```python
from build123d import *
from build123d.topology import SkipClean

# Parameters (mm, degrees)
BOSS_EXTRUDE1_DEPTH       = 1
BOSS_EXTRUDE1_DEPTH_BACK  = 1
SKETCH1_R                 = 5
SKETCH1_R_2               = 0.5
BOSS_EXTRUDE2_START       = -5.85
BOSS_EXTRUDE2_OUTLINE_W   = 15
BOSS_EXTRUDE2_OUTLINE_H   = 4
BOSS_EXTRUDE2_DEPTH       = 3
BOSS_EXTRUDE2_START_2     = -4
BOSS_EXTRUDE2_2_OUTLINE_R = 0.5
BOSS_EXTRUDE2_2_DEPTH     = 6
CUT_EXTRUDE4_DEPTH        = 8
SKETCH6_R                 = 0.8
CUT_EXTRUDE3_DEPTH        = 9
SKETCH9_W                 = 8
SKETCH9_H                 = 0.25
CUT_EXTRUDE5_DEPTH        = 2
SKETCH10_R                = 2.1
SKETCH10_R_2              = 0.8
CUT_EXTRUDE6_DEPTH        = 1.5
FILLET2_R                 = 1
FILLET3_START             = -5.85
FILLET3_DEPTH             = 1.5
CUT_EXTRUDE2_START        = -10
CUT_EXTRUDE2_DEPTH        = 10
BOSS_EXTRUDE3_START       = -2
BOSS_EXTRUDE3_DEPTH       = 2
FILLET4_R                 = 0.5
CUT_EXTRUDE7_DEPTH        = 1.5


with BuildPart() as part:
    # Sketch1 → Boss-Extrude1 (new, two sides: drawn at the far end of the back side and taken through both)
    with BuildSketch(Plane.XY.offset(-BOSS_EXTRUDE1_DEPTH_BACK)):
        Circle(SKETCH1_R)
        with Locations((-2.5, 1.095)):
            Circle(SKETCH1_R_2, mode=Mode.SUBTRACT)
        with Locations((2.5, 1.095)):
            Circle(SKETCH1_R_2, mode=Mode.SUBTRACT)
        with Locations((-2.5, -1.095)):
            Circle(SKETCH1_R_2, mode=Mode.SUBTRACT)
        with Locations((2.5, -1.095)):
            Circle(SKETCH1_R_2, mode=Mode.SUBTRACT)
        with Locations((-1.35, 2.5)):
            Circle(SKETCH1_R_2, mode=Mode.SUBTRACT)
        with Locations((-1.35, -2.5)):
            Circle(SKETCH1_R_2, mode=Mode.SUBTRACT)
    extrude(amount=BOSS_EXTRUDE1_DEPTH + BOSS_EXTRUDE1_DEPTH_BACK)

    # Boss-Extrude2: read off the stored shape, not the designer's step
    # Boss-Extrude2 outline → Boss-Extrude2 (add)
    with BuildSketch(Plane.YZ.offset(BOSS_EXTRUDE2_START)):
        with Locations((0, -1)):
            Rectangle(BOSS_EXTRUDE2_OUTLINE_W, BOSS_EXTRUDE2_OUTLINE_H)
    extrude(amount=BOSS_EXTRUDE2_DEPTH)

    # Boss-Extrude2 2 outline → Boss-Extrude2 2 (cut)
    with SkipClean():  # the faces are left unmerged after this step: merging them gives an invalid solid
        with BuildSketch(Plane.XY.offset(BOSS_EXTRUDE2_START_2)):
            with Locations((-2.5, 1.095)):
                Circle(BOSS_EXTRUDE2_2_OUTLINE_R)
            with Locations((-2.5, -1.095)):
                Circle(BOSS_EXTRUDE2_2_OUTLINE_R)
        extrude(amount=BOSS_EXTRUDE2_2_DEPTH, mode=Mode.SUBTRACT)

    # Sketch7 → Cut-Extrude4 (cut)
    with SkipClean():  # the faces are left unmerged after this step: merging them gives an invalid solid
        with BuildSketch(Plane(origin=(-2.85, 0, 0), x_dir=(0, 0, -1), z_dir=(1, 0, 0))):
            Polygon((-1, 7.5), (-1, 4.10822346), (1, 4.10822346), (1, 1.452071421), (3, 1.452071421), (3, 7.5), align=None)
            Polygon((-1, -4.10822346), (-1, -7.5), (3, -7.5), (3, -1.452071421), (1, -1.452071421), (1, -4.10822346), align=None)
        extrude(amount=CUT_EXTRUDE4_DEPTH, mode=Mode.SUBTRACT)

    # Sketch6 → Cut-Extrude3 (cut)
    with SkipClean():  # the faces are left unmerged after this step: merging them gives an invalid solid
        with BuildSketch(Plane.ZY.offset(5.85)):
            with Locations(Location((-1, 5.5, 0), (0, 0, 270))):
                Circle(SKETCH6_R)
            with Locations(Location((-1, -5.5, 0), (0, 0, 270))):
                Circle(SKETCH6_R)
        extrude(amount=-CUT_EXTRUDE3_DEPTH, mode=Mode.SUBTRACT)

    # Sketch9 → Cut-Extrude5 (cut)
    with SkipClean():  # the faces are left unmerged after this step: merging them gives an invalid solid
        with BuildSketch(Plane.XY.offset(1)):
            with Locations((1.15, 3.98322346)):
                Rectangle(SKETCH9_W, SKETCH9_H)
            with Locations((1.15, -3.98322346)):
                Rectangle(SKETCH9_W, SKETCH9_H)
        extrude(amount=-CUT_EXTRUDE5_DEPTH, mode=Mode.SUBTRACT)

    # Sketch10 → Cut-Extrude6 (cut)
    # profile 1 of 2: a face of its own
    with SkipClean():  # the faces are left unmerged after this step: merging them gives an invalid solid
        with BuildSketch(Plane.ZY.offset(5.85)):
            with Locations((-1, 5.5)):
                Circle(SKETCH10_R)
            with Locations((-1, 5.5)):
                Circle(SKETCH10_R_2, mode=Mode.SUBTRACT)
        # profile 2 of 2: a face of its own
        with BuildSketch(Plane.ZY.offset(5.85)):
            with Locations((-1, -5.5)):
                Circle(SKETCH10_R)
            with Locations((-1, -5.5)):
                Circle(SKETCH10_R_2, mode=Mode.SUBTRACT)
        extrude(amount=-CUT_EXTRUDE6_DEPTH, mode=Mode.SUBTRACT)

    # Fillet2
    fillet2_edges = [part.edges().sort_by_distance(p)[0] for p in [
        (-4.35, 7.5, -3),
        (-4.35, -7.5, 1),
        (-4.35, -7.5, -3),
        (-4.35, 7.5, 1),
    ]]
    fillet(fillet2_edges, radius=FILLET2_R)

    # Fillet3: read off the stored shape, not the designer's step
    # Fillet3 outline → Fillet3 (cut)
    with SkipClean():  # the faces are left unmerged after this step: merging them gives an invalid solid
        with BuildSketch(Plane.YZ.offset(FILLET3_START)):
            with BuildLine():
                ThreePointArc((-6.696065005, -2.726102113), (-6.574273302, -2.846043449), (-6.5, -3))
                Line((-6.5, -3), (-6.140312424, -3))
                ThreePointArc((-6.140312424, -3), (-6.428345587, -2.883659861), (-6.696065005, -2.726102113))
            make_face()
            with BuildLine():
                ThreePointArc((-7.5, -2), (-7.346043449, -2.074273302), (-7.226102113, -2.196065005))
                ThreePointArc((-7.226102113, -2.196065005), (-7.383659861, -1.928345587), (-7.5, -1.640312424))
                Line((-7.5, -1.640312424), (-7.5, -2))
            make_face()
            with BuildLine():
                ThreePointArc((-3.784723184, -2.211538462), (-4.257978234, -2.693334561), (-4.859687576, -3))
                Line((-4.859687576, -3), (-3.376323942, -3))
                ThreePointArc((-3.376323942, -3), (-3.820300726, -2.729966553), (-3.784723184, -2.211538462))
            make_face()
            with BuildLine():
                Line((-7.5, 0), (-7.5, -0.359687576))
                ThreePointArc((-7.5, -0.359687576), (-7.383659861, -0.071654413), (-7.226102112, 0.196065005))
                ThreePointArc((-7.226102112, 0.196065005), (-7.346043449, 0.074273302), (-7.5, 0))
            make_face()
            with BuildLine():
                ThreePointArc((-4.859687576, 1), (-4.257978234, 0.693334561), (-3.784723184, 0.211538462))
                ThreePointArc((-3.784723184, 0.211538462), (-3.820300726, 0.729966553), (-3.376323942, 1))
                Line((-3.376323942, 1), (-4.859687576, 1))
            make_face()
            with BuildLine():
                ThreePointArc((3.784723184, -2.211538462), (3.820300726, -2.729966553), (3.376323942, -3))
                Line((3.376323942, -3), (4.859687576, -3))
                ThreePointArc((4.859687576, -3), (4.257978234, -2.693334561), (3.784723184, -2.211538462))
            make_face()
            with BuildLine():
                ThreePointArc((-6.5, 1), (-6.574273302, 0.846043449), (-6.696065005, 0.726102113))
                ThreePointArc((-6.696065005, 0.726102113), (-6.428345587, 0.883659861), (-6.140312424, 1))
                Line((-6.140312424, 1), (-6.5, 1))
            make_face()
            with BuildLine():
                Line((4.859687576, 1), (3.376323942, 1))
                ThreePointArc((3.376323942, 1), (3.820300726, 0.729966553), (3.784723184, 0.211538462))
                ThreePointArc((3.784723184, 0.211538462), (4.257978234, 0.693334561), (4.859687576, 1))
            make_face()
            with BuildLine():
                ThreePointArc((6.696065005, -2.726102112), (6.428345587, -2.883659861), (6.140312424, -3))
                Line((6.140312424, -3), (6.5, -3))
                ThreePointArc((6.5, -3), (6.574273302, -2.846043449), (6.696065005, -2.726102112))
            make_face()
            with BuildLine():
                Line((6.5, 1), (6.140312424, 1))
                ThreePointArc((6.140312424, 1), (6.428345587, 0.883659861), (6.696065005, 0.726102112))
                ThreePointArc((6.696065005, 0.726102112), (6.574273302, 0.846043449), (6.5, 1))
            make_face()
            with BuildLine():
                ThreePointArc((7.5, -1.640312424), (7.383659861, -1.928345587), (7.226102112, -2.196065005))
                ThreePointArc((7.226102112, -2.196065005), (7.346043449, -2.074273302), (7.5, -2))
                Line((7.5, -2), (7.5, -1.640312424))
            make_face()
            with BuildLine():
                ThreePointArc((7.5, 0), (7.346043449, 0.074273302), (7.226102113, 0.196065005))
                ThreePointArc((7.226102113, 0.196065005), (7.383659861, -0.071654413), (7.5, -0.359687576))
                Line((7.5, -0.359687576), (7.5, 0))
            make_face()
        extrude(amount=FILLET3_DEPTH, mode=Mode.SUBTRACT)

    # Sketch3 → Cut-Extrude2 (cut)
    with SkipClean():  # the faces are left unmerged after this step: merging them gives an invalid solid
        with BuildSketch(Plane.XY.offset(1).offset(CUT_EXTRUDE2_START)):
            with BuildLine():
                ThreePointArc((3.5, -3.570714214), (5, 0), (3.5, 3.570714214))
                Line((3.5, 3.570714214), (3.5, -3.570714214))
            make_face()
        extrude(amount=CUT_EXTRUDE2_DEPTH, mode=Mode.SUBTRACT)

    # Sketch11 → Boss-Extrude3 (add)
    with SkipClean():  # the faces are left unmerged after this step: merging them gives an invalid solid
        with BuildSketch(Plane.XY.offset(1).offset(BOSS_EXTRUDE3_START)):
            with BuildLine():
                Line((0, -3.85822346), (0, -5))
                ThreePointArc((0, -5), (1.689509204, -4.705906783), (3.180269129, -3.85822346))
                Line((3.180269129, -3.85822346), (0, -3.85822346))
            make_face()
            with BuildLine():
                Line((0, 5), (0, 3.85822346))
                Line((0, 3.85822346), (3.180269129, 3.85822346))
                ThreePointArc((3.180269129, 3.85822346), (1.689509204, 4.705906783), (0, 5))
            make_face()
        extrude(amount=BOSS_EXTRUDE3_DEPTH)

    # Fillet4
    fillet4_edges = [part.edges().sort_by_distance(p)[0] for p in [
        (0, -5, 0),
        (0, -3.85822346, 0),
        (0, 3.85822346, 0),
        (0, 5, 0),
    ]]
    fillet(fillet4_edges, radius=FILLET4_R)

    # Sketch12 → Cut-Extrude7 (cut)
    with BuildSketch(Plane.ZY.offset(5.85)):
        with BuildLine():
            ThreePointArc((1, 6.5), (0.707106781, 7.207106781), (0, 7.5))
            ThreePointArc((0, 7.5), (0.074273302, 7.346043449), (0.196065005, 7.226102113))
            ThreePointArc((0.196065005, 7.226102113), (0.48492424, 6.98492424), (0.726102113, 6.696065005))
            ThreePointArc((0.726102113, 6.696065005), (0.846043449, 6.574273302), (1, 6.5))
        make_face()
        with BuildLine():
            ThreePointArc((-2.726102113, -6.696065005), (-2.48492424, -6.98492424), (-2.196065005, -7.226102113))
            ThreePointArc((-2.196065005, -7.226102113), (-2.074273302, -7.346043449), (-2, -7.5))
            ThreePointArc((-2, -7.5), (-2.707106781, -7.207106781), (-3, -6.5))
            ThreePointArc((-3, -6.5), (-2.846043449, -6.574273302), (-2.726102113, -6.696065005))
        make_face()
        with BuildLine():
            ThreePointArc((0, -7.5), (0.707106781, -7.207106781), (1, -6.5))
            ThreePointArc((1, -6.5), (0.846043449, -6.574273302), (0.726102113, -6.696065005))
            ThreePointArc((0.726102113, -6.696065005), (0.48492424, -6.98492424), (0.196065005, -7.226102113))
            ThreePointArc((0.196065005, -7.226102113), (0.074273302, -7.346043449), (0, -7.5))
        make_face()
        with BuildLine():
            ThreePointArc((-2, 7.5), (-2.707106781, 7.207106781), (-3, 6.5))
            ThreePointArc((-3, 6.5), (-2.846043449, 6.574273302), (-2.726102113, 6.696065005))
            ThreePointArc((-2.726102113, 6.696065005), (-2.48492424, 6.98492424), (-2.196065005, 7.226102113))
            ThreePointArc((-2.196065005, 7.226102113), (-2.074273302, 7.346043449), (-2, 7.5))
        make_face()
    extrude(amount=-CUT_EXTRUDE7_DEPTH, mode=Mode.SUBTRACT)


solid = part.part
```
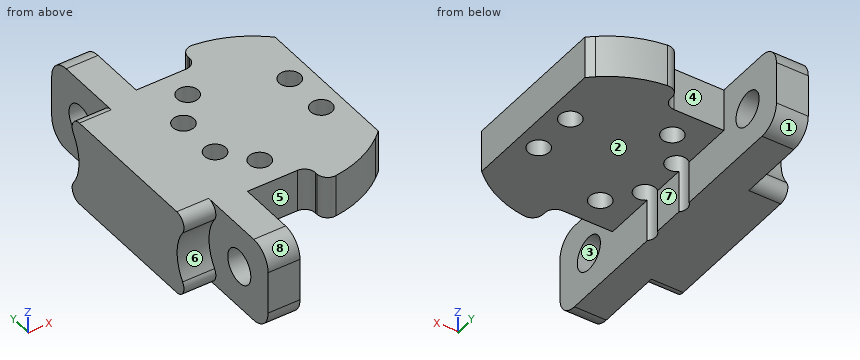
Source: CAD feature listing. Evaluate the final solid. Frame: model axes, mm. Face numbers are marked on the shaded views. A direction names the side the tool comes from. Give positions to 0.01 mm unless a question says otherwise; leave off trailing zeros. Loops run counter-clockwise (first coordinate to the right, second up) from the corner with the lowest first, then second, coordinate; pieces in that order, holes last. Notation, with made-up numbers: (-6.75, 42) -> (14.25, 42) arc R12 cw to (14.25, 47) -> close; hole circle Ø8 at (85.25, 42.25). An arc over 180 degrees is marked (long way). Put each result on its own line as item: value. Start each with the question number.
1) Material intervals for probe 1 along Y at (x, z) = (2.5, -0.5) (3 decimals); probe 2 along X at (y, z) = (6.75, -1.1); probe 3 along Z at (x, y) = (1.5, -3), sorted ascending.
2) Cut plane B-B (y = -2.5). Return loops of the section in (x, z), then the cut area to 3 significant figures.
3) Cut plane C-C (x = -4). Return loops of the section in (y, z).
4) Cut plane D-D (z = -0.8). State how many separate pieces and enclosed holes the cut face has, then the cut area to 3 significant figures.
5) Cut plane A-A (x = -2.5). Return loops of the section in (y, z) (3 decimals), then the cut area to 3 significant figures.
6) Reachability of the marked faces 4, 5, 6, 7 and 8 from +Z, -Z, +X, -X, +Y, -Y: full face, straight path, thin tool, end or side. Return the list, or none.
7) Draft query along Y for the marked faces 1, 2 and 3. Return one class per face: released by +Y, released by -Y, zero draft, split by the parting line, or undercut.
8) Contact query for flat-ended pins moving along their axis: P1, Ø1, axis at x = -1, z = 0, coming from the -Y side; P2, Ø0.7, axis at y = 0, z = -2, coming from the +X side; P3, Ø2, axis at y = 5.5, z = -1.5, coming from the -X side; P4, Ø1.5, axis at x = -4.5, z = 0, coming from the +Y side. Output: stop coordinate, or through.
Results are:
1. probe 1: y = -4.33 to -1.595, -0.595 to 0.595, 1.595 to 4.33
1. probe 2: x = -4.35 to -2.85
1. probe 3: z = -1 to 1
2. outline: (-5.85, -3) -> (-2.85, -3) -> (-2.85, -1) -> (-1.85, -1) -> (-1.85, 1) -> (-5.85, 1) -> close; (-0.85, -1) -> (3.5, -1) -> (3.5, 1) -> (-0.85, 1) -> close
2. area: 22.7 mm2
3. outline: (-7.5, -2) arc R1 ccw to (-6.5, -3) -> (6.5, -3) arc R1 ccw to (7.5, -2) -> (7.5, 0) arc R1 ccw to (6.5, 1) -> (-6.5, 1) arc R1 ccw to (-7.5, 0) -> close; hole circle Ø1.6 at (-5.5, -1); hole circle Ø1.6 at (5.5, -1)
4. separate pieces: 3
4. enclosed holes: 6
4. area: 77.2 mm2
5. outline: (-3.858, -1) -> (-1.595, -1) -> (-1.595, 1) -> (-3.858, 1) -> close; (-0.595, -1) -> (0.595, -1) -> (0.595, 1) -> (-0.595, 1) -> close; (1.595, -1) -> (3.858, -1) -> (3.858, 1) -> (1.595, 1) -> close
5. area: 11.4 mm2
6. face 4: +Z, -Z, +Y
6. face 5: +Z, -Z, -Y
6. face 6: -X, -Y
6. face 7: -Z, +X, +Y, -Y
6. face 8: +Z, +X, -X, -Y
7. face 1: released by +Y
7. face 2: zero draft
7. face 3: undercut
8. P1: stops at y = -3.86
8. P2: stops at x = -2.85
8. P3: stops at x = -4.35
8. P4: stops at y = 7.5
